The model under review builds one solid part; all positions refer to its coordinate system, in mm. Face numbers are marked on the shaded views. A direction names the side the tool comes from. Give positions to 0.01 mm unless a question says otherwise; leave off trailing zeros. Write each loop counter-clockwise with the first axis right and the second up, starting at its lowest first coordinate (ties: lowest second). Pieces come first, ordered by that corner, then holes. Notation, with made-up numbers: (37, -27.75) - (82, -27.75) arc R25 ccw to (82, -2.75) - close; hole circle Ø9 at (74, 14). An arc over 180 degrees is marked (long way). Write item = value, one per line.
```python
from build123d import *

# Parameters (mm, degrees)
F0_W     = 30
F0_H     = 30
F1_DEPTH = 10
F2_R     = 10
F3_DEPTH = 10
F5_D     = 5.25


with BuildPart() as f1:
    # F0 (on Front) → F1 (new body, symmetric)
    with BuildSketch(Plane.XZ):
        Rectangle(F0_W, F0_H)
    extrude(amount=F1_DEPTH, both=True)

    # F2 (on face) → F3 (cut)
    with BuildSketch(Plane.XZ.offset(10)):
        Circle(F2_R)
    extrude(amount=-F3_DEPTH, mode=Mode.SUBTRACT)

    # F5 (through all)
    with Locations(Plane(origin=(0, 10, 0), x_dir=(-1, 0, 0), z_dir=(0, 1, 0))):
        with Locations((0, 0)):
            Hole(F5_D / 2)


solid = f1.part
```
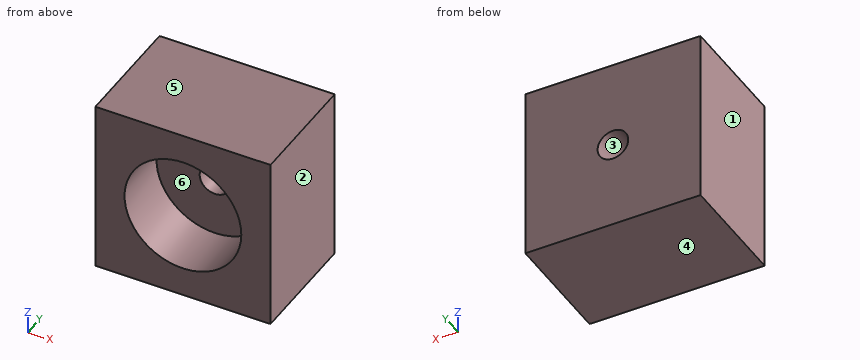
1. Draft analysis for pull direction X (two halves, no side actions). For the marked faces 1, 2, 3 and 4, state which applies: +X half, -X half, draft (parallel to the pull), parting line (faces both ways), or undercut.
Findings below:
face_1 = -X half
face_2 = +X half
face_3 = undercut
face_4 = draft
2. Take a section at C-C on y = -7.75. Give the boundary of the cut face in (x, z), and give its area (3 significant figures).
Findings below:
outline = (-15, -15) - (15, -15) - (15, 15) - (-15, 15) - close; hole circle Ø20 at (0, 0)
area = 586 mm²
3. For line 1 (Z direction, x = 0, y = 2.5) (3 decimals); line 2 (Z direction, x = 0, y = -6.75); line 3 (Y direction, x = 5.5, z = 4.75), list the stretches that pass through material, from the lowest coordinate up. Write a range as from..to.
Findings below:
line_1 = -15..-2.625, 2.625..15
line_2 = -15..-10, 10..15
line_3 = 0..10
4. Insertion check: P1, Ø4, axis at x = 0, z = 0, coming from the -Y side; P2, Ø12, axis at x = 0, z = 0, coming from the -Y side. Each pin has a flat end and moves straight along its axis. Give the tip position at first contact, or say it passes through.
Findings below:
P1 = through
P2 = 0
5. Take a section at A-A on z = 0. Give the boundary of the cut face in (x, y) (3 decimals), and give its area (4 significant figures).
Findings below:
outline = (-15, -10) - (-10, -10) - (-10, 0) - (-2.625, 0) - (-2.625, 10) - (-15, 10) - close; (2.625, 0) - (10, 0) - (10, -10) - (15, -10) - (15, 10) - (2.625, 10) - close
area = 347.5 mm²
6. Machinability: for the marked faces 5 and 6, which of the approach directions +Z, -Z, +X, -X, +Y, -Y give a long, thin tool a straight path to every point of the face, cutting with its end or side? Answer none if there is none.
Findings below:
face_5 = +Z, +X, -X, +Y, -Y
face_6 = -Y
7. Take a section at B-B on x = 0. Give the boundary of the cut face in (y, z) (3 decimals).
Findings below:
outline = (-10, -15) - (10, -15) - (10, -2.625) - (0, -2.625) - (0, -10) - (-10, -10) - close; (-10, 10) - (0, 10) - (0, 2.625) - (10, 2.625) - (10, 15) - (-10, 15) - close
8. Take a section at D-D on z = 7.25. Give the boundary of the cut face in (x, y), and give its area (3 significant figures).
Findings below:
outline = (-15, -10) - (-6.89, -10) - (-6.89, 0) - (6.89, 0) - (6.89, -10) - (15, -10) - (15, 10) - (-15, 10) - close
area = 462 mm²
